Can you work these out from the model? Positions are in its coordinate system, mm. Face numbers are marked on the shaded views. Coordinates: 2 decimals unless noted, no trailing zeros. Order: outer loops, then holes, each group sorted by start corner. A loop starts at its lowest first (then second) coordinate and runs counter-clockwise, first axis right, second up. Notation, with made-up numbers: (51, 43) - (79, 43) arc R10 ccw to (79, 54) - close; hole circle Ø10 at (22.25, -11.5). An arc over 180 degrees is marked (long way). Use a Markdown table: item, result. Add a question column.
(1) We'd pull the mould along Y, two halves only. Please class the marked faces 1, 2 and 3: pulls with the +Y half, pulls with the -Y half, needs draft (parallel to the pull), parting line crosses it, or undercut.
(2) I want a section at D-D (y = -31). List the corners of the cut face in (x, z) for me.
(3) For pin 1 Ø13 at (x, y) = (66.12, -17.2) entering from +Z, with a flat end and sliding along its axis, tell me the tip position at first contact or that it passes through.
(4) I want a section at B-B (y = -13.5). List the corners of the cut face in (x, z) for me.
(5) I want a section at A-A (x = 48). List the corners of the cut face in (y, z) for me.
(6) If I drill on L1, parallel to X at y = -17.5, z = -2.95; L2, parallel to X at y = -9.5, z = 1.3; L3, parallel to Y at x = 44.5, z = -0.45, over which ranges is the centre line in solid material (lowest first)? Write a range as [from, to].
(7) I want a section at C-C (z = -2.5). List the corners of the cut face in (x, y) for me (3 decimals).
```python
from build123d import *

# Parameters (mm, degrees)
F1_DEPTH = 3.302
F2_DEPTH = 2.54
F3_R     = 5.715
F3_W     = 9.652
F3_H     = 4.445
F3_H_2   = 8.255
F4_DEPTH = 3.303


with BuildPart() as f1:
    # F0 (on Top) → F1 (new body)
    with BuildSketch(Plane.XY):
        with BuildLine():
            Line((86.51892, -3.862933), (10.31892, -3.862933))
            ThreePointArc((10.31892, -3.862933), (8.073856, -4.792869), (7.14392, -7.037933))
            Line((7.14392, -7.037933), (7.14392, -32.437933))
            ThreePointArc((7.14392, -32.437933), (8.073856, -34.682997), (10.31892, -35.612933))
            Line((10.31892, -35.612933), (86.51892, -35.612933))
            ThreePointArc((86.51892, -35.612933), (88.763984, -34.682997), (89.69392, -32.437933))
            Line((89.69392, -32.437933), (89.69392, -7.037933))
            ThreePointArc((89.69392, -7.037933), (88.763984, -4.792869), (86.51892, -3.862933))
        make_face()
        with BuildLine():
            Line((83.97892, -33.072933), (12.85892, -33.072933))
            ThreePointArc((12.85892, -33.072933), (10.613856, -32.142997), (9.68392, -29.897933))
            Line((9.68392, -29.897933), (9.68392, -9.577933))
            ThreePointArc((9.68392, -9.577933), (10.613856, -7.332869), (12.85892, -6.402933))
            Line((12.85892, -6.402933), (83.97892, -6.402933))
            ThreePointArc((83.97892, -6.402933), (86.223984, -7.332869), (87.15392, -9.577933))
            Line((87.15392, -9.577933), (87.15392, -29.897933))
            ThreePointArc((87.15392, -29.897933), (86.223984, -32.142997), (83.97892, -33.072933))
        make_face(mode=Mode.SUBTRACT)
        with BuildLine():
            ThreePointArc((9.68392, -29.897933), (10.613856, -32.142997), (12.85892, -33.072933))
            Line((12.85892, -33.072933), (83.97892, -33.072933))
            ThreePointArc((83.97892, -33.072933), (86.223984, -32.142997), (87.15392, -29.897933))
            Line((87.15392, -29.897933), (87.15392, -9.577933))
            ThreePointArc((87.15392, -9.577933), (86.223984, -7.332869), (83.97892, -6.402933))
            Line((83.97892, -6.402933), (12.85892, -6.402933))
            ThreePointArc((12.85892, -6.402933), (10.613856, -7.332869), (9.68392, -9.577933))
            Line((9.68392, -9.577933), (9.68392, -29.897933))
        make_face()
    extrude(amount=-F1_DEPTH)

    # F0 (on Top) → F2 (join)
    with BuildSketch(Plane.XY):
        with BuildLine():
            Line((86.51892, -3.862933), (10.31892, -3.862933))
            ThreePointArc((10.31892, -3.862933), (8.073856, -4.792869), (7.14392, -7.037933))
            Line((7.14392, -7.037933), (7.14392, -32.437933))
            ThreePointArc((7.14392, -32.437933), (8.073856, -34.682997), (10.31892, -35.612933))
            Line((10.31892, -35.612933), (86.51892, -35.612933))
            ThreePointArc((86.51892, -35.612933), (88.763984, -34.682997), (89.69392, -32.437933))
            Line((89.69392, -32.437933), (89.69392, -7.037933))
            ThreePointArc((89.69392, -7.037933), (88.763984, -4.792869), (86.51892, -3.862933))
        make_face()
        with BuildLine():
            Line((83.97892, -33.072933), (12.85892, -33.072933))
            ThreePointArc((12.85892, -33.072933), (10.613856, -32.142997), (9.68392, -29.897933))
            Line((9.68392, -29.897933), (9.68392, -9.577933))
            ThreePointArc((9.68392, -9.577933), (10.613856, -7.332869), (12.85892, -6.402933))
            Line((12.85892, -6.402933), (83.97892, -6.402933))
            ThreePointArc((83.97892, -6.402933), (86.223984, -7.332869), (87.15392, -9.577933))
            Line((87.15392, -9.577933), (87.15392, -29.897933))
            ThreePointArc((87.15392, -29.897933), (86.223984, -32.142997), (83.97892, -33.072933))
        make_face(mode=Mode.SUBTRACT)
    extrude(amount=F2_DEPTH)

    # F3 (on Top) → F4 (cut, through all)
    with BuildSketch(Plane.XY):
        with Locations((30.71512, -17.197933)):
            Circle(F3_R)
        with BuildLine():
            ThreePointArc((71.83772, -17.197933), (66.12272, -11.482933), (60.40772, -17.197933))
            ThreePointArc((60.40772, -17.197933), (66.12272, -22.912933), (71.83772, -17.197933))
        make_face()
        with Locations((48.41892, -14.975433)):
            Rectangle(F3_W, F3_H)
        with Locations((48.41892, -21.325433)):
            Rectangle(F3_W, F3_H_2)
    extrude(amount=-F4_DEPTH, mode=Mode.SUBTRACT)


solid = f1.part
```
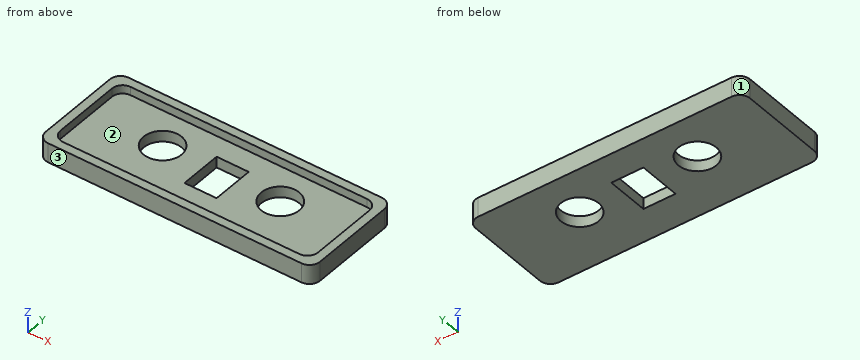
Answers follow:
| question | item | result |
|---|---|---|
| 1 | face 1 | pulls with the +Y half |
| 1 | face 2 | undercut |
| 1 | face 3 | pulls with the -Y half |
| 2 | outline | (7.14, -3.3) - (89.69, -3.3) - (89.69, 2.54) - (86.96, 2.54) - (86.96, 0) - (9.88, 0) - (9.88, 2.54) - (7.14, 2.54) - close |
| 3 | pin 1 | stops at z = 0 |
| 4 | outline | (7.14, -3.3) - (26.36, -3.3) - (26.36, 0) - (9.68, 0) - (9.68, 2.54) - (7.14, 2.54) - close; (35.07, -3.3) - (43.59, -3.3) - (43.59, 0) - (35.07, 0) - close; (53.24, -3.3) - (61.77, -3.3) - (61.77, 0) - (53.24, 0) - close; (70.48, -3.3) - (89.69, -3.3) - (89.69, 2.54) - (87.15, 2.54) - (87.15, 0) - (70.48, 0) - close |
| 5 | outline | (-35.61, -3.3) - (-25.45, -3.3) - (-25.45, 0) - (-33.07, 0) - (-33.07, 2.54) - (-35.61, 2.54) - close; (-12.75, -3.3) - (-3.86, -3.3) - (-3.86, 2.54) - (-6.4, 2.54) - (-6.4, 0) - (-12.75, 0) - close |
| 6 | L1 | x = [7.14, 25.01], [36.42, 43.59], [53.24, 60.42], [71.83, 89.69] |
| 6 | L2 | x = [7.14, 9.68], [87.15, 89.69] |
| 6 | L3 | y = [-35.61, -25.45], [-12.75, -3.86] |
| 7 | outline | (7.144, -32.438) arc R3.175 ccw to (10.319, -35.613) - (86.519, -35.613) arc R3.175 ccw to (89.694, -32.438) - (89.694, -7.038) arc R3.175 ccw to (86.519, -3.863) - (10.319, -3.863) arc R3.175 ccw to (7.144, -7.038) - close; hole circle Ø11.43 at (30.715, -17.198); hole (43.593, -25.453) - (53.245, -25.453) - (53.245, -12.753) - (43.593, -12.753) - close; hole circle Ø11.43 at (66.123, -17.198) |
